Autodesk Inventor part; units mm, degrees
ref_plane "Work Plane1" through (-7.9612, 0, 0) normal (0, -0.866, -0.5) x (1, 0, 0)
ref_plane "YZ Plane" through (0, 0, 0) normal (1, 0, 0) x (0, 1, 0)
ref_plane "XZ Plane" through (0, 0, 0) normal (0, 1, 0) x (-1, 0, 0)
sketch "Esquisse1" plane through (0, 0, 0) normal (1, 0, 0) x (0, 1, 0)
  line L0 (-4.0415, 0) -> (-2.0207, 3.5)
  line L1 (-2.0207, 3.5) -> (2.0207, 3.5)
  line L2 (2.0207, 3.5) -> (4.0415, 0)
  line L3 (4.0415, 0) -> (2.0207, -3.5)
  line L4 (2.0207, -3.5) -> (-2.0207, -3.5)
  line L5 (-2.0207, -3.5) -> (-4.0415, 0)
  point P0 (0, 0)
  point P1 (0, 0)
  dimension "d0" = 8.0829
extrude "Corps" add sketch "Esquisse1" along normal blind 3.2
sketch "Esquisse2" plane through (0, 0, 0) normal (0, 0, 1) x (1, 0, 0)
  line L0 (0, 2.0207) -> (0, 4.0415)
  line L1 (0, 4.0415) -> (3.2, 4.0415)
  line L2 (3.2, 2.0207) -> (3.2, 4.0415)
  line L3 (-0.64, 0) -> (3.84, 0)
  line L4 (0.659, 4.0415) -> (0, 2.9)
  line L5 (2.541, 4.0415) -> (3.2, 2.9)
  dimension "d3" = 30
  dimension "d4" = 30
  dimension "d5" = 5.8
  dimension "d6" = 5.8
revolve "Chanfrein1" cut sketch "Esquisse2" angle 360 about axis through (-10, 0, 0) along (1, 0, 0)
sketch "Esquisse3" plane through (3.2, 0, 0) normal (1, 0, 0) x (0, 0, -1)
  arc A0 (-0.625, -1.0825) -> (0.625, -1.0825) centre (0, 0) ccw
hole "Filetage" at (3.2, 0, 0) direction (-1, 0, 0) diameter 3.242 end through all
chamfer "Chanfrein2" distance 0.3789 angle 30 1 edges at (3.2, 0, 1.621) measured on face at (3.2, 2.4416, -0.2965)
chamfer "Chanfrein3" distance 0.3789 angle 30 1 edges at (0, 0, 1.621) measured on face at (0, 2.4416, -0.2965)
ref_plane "Work Plane1" through (-7.9612, 0, 0) normal (0, -0.866, -0.5) x (1, 0, 0)
equation "\"d0\" = 1.1547 * SW"
equation "\"d1\" = KOH"
equation "\"d3\" = ANG1"
equation "\"d4\" = ANG2"
equation "\"d5\" = SW0"
equation "\"d6\" = SW01"
equation "\"d8\" = -0.5 * GD1 + 0.5 * NND"
equation "\"d40\" = -0.5 * GD1 + 0.5 * NND"
equation "\"d10\" = -0.5 * GD1 + 0.5 * NND"
equation "\"d41\" = -0.5 * GD1 + 0.5 * NND"
equation "\"ANG1\" = 30deg"
equation "\"ANG2\" = 30deg"
equation "\"NND\" = 4"
equation "\"KOH\" = 3.2"
equation "\"SW\" = 7"
equation "\"SW0\" = SW01"
equation "\"SW01\" = 5.8"
equation "\"GUL\" = 0.541266 * PTC"
equation "\"THREADDIA\" = 4"
equation "\"TOA\" = 30deg"
equation "\"PTC\" = 0.7"
equation "\"E0\" = 1.155 * SW"
equation "\"GAL\" = 0.541266 * PTC"
properties part number "DIN 934 - M4" material "Acier, doux"
Here's how the part is built. I have some questions about the finished solid (model axes, mm). Coordinates: 2 decimals unless noted, no trailing zeros. Write each loop counter-clockwise with the first axis right and the second up, starting at its lowest first coordinate (ties: lowest second). Pieces come first, ordered by that corner, then holes. Notation, with made-up numbers: M 22.25,-13 L 39.25,-13 A20 cw 39.25,13 Z; hole C 49,52 d8. An arc over 180 degrees is marked long. Answer as CSV lines item,"result". Start each with the question number.
Q1. I need wall thicknesses on probe 1 along Z at (x, y) = (1.3, 0); probe 2 along Y at (x, z) = (2.45, 0.25); probe 3 along Z at (x, y) = (1.7, -3). Which ranges of each line are inside material? Lowest first, please. Write a range as [from, to].
Q2. Suppose I cut it at C-C, the plane x = 0.5. List the corners of the cut face in (y, z) for me, then the cut area to 3 significant figures.
Q3. Suppose I cut it at A-A, the plane y = 0. List the corners of the cut face in (x, z) for me, then the cut area to 3 significant figures.
Q4. Suppose I cut it at B-B, the plane x = 1.8. List the corners of the cut face in (y, z) for me.
Q5. If we mould it in two halves opening along Y, with no side actions, what happens to faces 1 (the flat face through (1.6, -3, -1.8)), 2 (the flat face through (3.2, 2, 1)), 3 (the cylindrical face through (1.581, 1.438, -0.748))? For each: pulls with the +Y half, pulls with the -Y half, needs draft (parallel to the pull), parting line crosses it, or undercut.
Entries:
1,probe 1,"z = [-3.5, -1.62], [1.62, 3.5]"
1,probe 2,"y = [-3.9, -1.6], [1.6, 3.9]"
1,probe 3,"z = [-1.8, 1.8]"
2,outline,"M -3.73,-0.55 L -2.34,-2.95 A3.77 ccw -1.39,-3.5 L 1.39,-3.5 A3.77 ccw 2.34,-2.95 L 3.73,-0.55 A3.77 ccw 3.73,0.55 L 2.34,2.95 A3.77 ccw 1.39,3.5 L -1.39,3.5 A3.77 ccw -2.34,2.95 L -3.73,0.55 A3.77 ccw Z; hole C 0,0 d3.24"
2,area,"33.3 mm²"
3,outline,"M 0,-2.9 L 0.35,-3.5 L 2.85,-3.5 L 3.2,-2.9 L 3.2,-2 L 2.98,-1.62 L 0.22,-1.62 L 0,-2 Z; M 0,2 L 0.22,1.62 L 2.98,1.62 L 3.2,2 L 3.2,2.9 L 2.85,3.5 L 0.35,3.5 L 0,2.9 Z"
3,area,"11.4 mm²"
4,outline,"M -4.04,0 L -2.02,-3.5 L 2.02,-3.5 L 4.04,0 L 2.02,3.5 L -2.02,3.5 Z; hole C 0,0 d3.24"
5,face 1,"pulls with the -Y half"
5,face 2,"needs draft"
5,face 3,"undercut"
